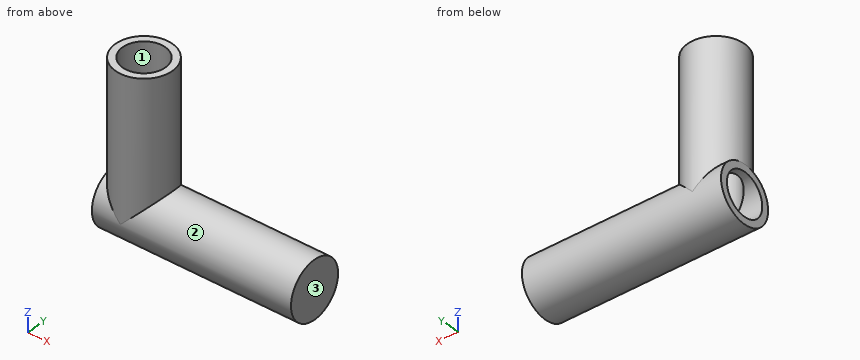
```python
from build123d import *

# Parameters (mm, degrees)
F0_R          = 10
F1_DEPTH      = 40
F1_DEPTH_BACK = 10
F2_R          = 10
F3_DEPTH      = 50
F3_DEPTH_BACK = 20
F4_R          = 7.5
F5_DEPTH      = 35
F5_DEPTH_BACK = 25
F6_R          = 7.5
F7_DEPTH      = 50


with BuildPart() as f1:
    # F0 (on Top) → F1 (new body, two sides)
    with BuildSketch(Plane.XY) as f1_sk:
        with Locations((-9.956808, 0)):
            Circle(F0_R)
    extrude(amount=F1_DEPTH)
    extrude(f1_sk.sketch, amount=-F1_DEPTH_BACK)

    # F2 (on Right) → F3 (join, two sides)
    with BuildSketch(Plane.YZ) as f3_sk:
        with Locations((0, -10)):
            Circle(F2_R)
    extrude(amount=F3_DEPTH)
    extrude(f3_sk.sketch, amount=-F3_DEPTH_BACK)

    # F4 (on Right) → F5 (cut, two sides)
    with BuildSketch(Plane.YZ) as f5_sk:
        with Locations((0, -10)):
            Circle(F4_R)
    extrude(amount=F5_DEPTH, mode=Mode.SUBTRACT)
    extrude(f5_sk.sketch, amount=-F5_DEPTH_BACK, mode=Mode.SUBTRACT)

    # F6 (on face) → F7 (cut)
    with BuildSketch(Plane.XY.offset(40)):
        with Locations((-9.956808, 0)):
            Circle(F6_R)
    extrude(amount=-F7_DEPTH, mode=Mode.SUBTRACT)


solid = f1.part
```
Model file for the job. Use its own axes, mm. Face numbers are marked on the shaded views. Give positions to 0.01 mm unless a question says otherwise; leave off trailing zeros. Loops run counter-clockwise (first coordinate to the right, second up) from the corner with the lowest first, then second, coordinate; pieces in that order, holes last. Notation, with made-up numbers: (50.5, 25) -> (88.5, 25) arc R18 ccw to (88.5, 32) -> close; hole circle Ø6 at (86, 79). An arc over 180 degrees is marked (long way). Write each question's results on one line, items separated by ' | '.
(1) Cut at D-D on y = -4.25. List the corners of the cut face in (x, z), and give its area (3 significant figures).
Geometry results:
outline: (-20, -19.05) -> (50, -19.05) -> (50, -0.95) -> (-0.9, -0.95) -> (-0.9, 40) -> (-3.78, 40) -> (-3.78, -3.82) -> (35, -3.82) -> (35, -16.18) -> (-20, -16.18) -> close; (-20, -3.82) -> (-16.14, -3.82) -> (-16.14, 40) -> (-19.01, 40) -> (-19.01, -0.95) -> (-20, -0.95) -> close | area: 787 mm²
(2) Probe line 1 along Z through (x, y) = (9, 0); line 2 along Y through (x, z) = (-15, -10); line 3 along X through (y, z) = (6, -13). List the from-to ranges inside material, lowest first.
Geometry results:
line 1: z = -20 to -17.5, -2.5 to 0 | line 2: y = -10 to -7.5, 7.5 to 10 | line 3: x = 35 to 50
(3) Pull direction Y, two halves, no side cores. Call the marked faces 1, 2 and 3: released by +Y, released by -Y, zero draft, split by the parting line, or undercut.
Geometry results:
face 1: undercut | face 2: split by the parting line | face 3: zero draft
(4) Cut at C-C on x = -11.5. List the corners of the cut face in (y, z).
Geometry results:
outline: (-9.88, -8.46) arc R10 ccw (long way) to (9.88, -8.46) -> (9.88, 40) -> (7.34, 40) -> (7.34, -8.46) arc R7.5 cw (long way) to (-7.34, -8.46) -> (-7.34, 40) -> (-9.88, 40) -> close
(5) Flat gauge pins, fed straight in: pin 1 Ø9 at (y, z) = (0, -10) entering from -X; pin 2 Ø12 at (x, y) = (13.5, -4.5) entering from -Z; pin 3 Ø3 at (x, y) = (19, 6.5) entering from -Z; pin 4 Ø6 at (y, z) = (-1.5, 5.5) entering from -X. Where does each tip first touch, or does it go through?
Geometry results:
pin 1: stops at x = 35 | pin 2: stops at z = -20 | pin 3: stops at z = -18.66 | pin 4: stops at x = -19.96
(6) Cut at B-B on z = -7.5. List the corners of the cut face in (x, y).
Geometry results:
outline: (-20, -9.68) -> (-12.46, -9.68) arc R10 ccw to (-7.46, -9.68) -> (50, -9.68) -> (50, 9.68) -> (-7.46, 9.68) arc R10 ccw to (-12.46, 9.68) -> (-20, 9.68) -> (-20, 7.07) -> (-12.46, 7.07) arc R7.5 cw to (-7.46, 7.07) -> (35, 7.07) -> (35, -7.07) -> (-7.46, -7.07) arc R7.5 cw to (-12.46, -7.07) -> (-20, -7.07) -> close
(7) Cut at A-A on y = 0. List the corners of the cut face in (x, z), and give its area (4 significant figures).
Geometry results:
outline: (-20, -20) -> (50, -20) -> (50, 0) -> (0.04, 0) -> (0.04, 40) -> (-2.46, 40) -> (-2.46, -2.5) -> (35, -2.5) -> (35, -17.5) -> (-20, -17.5) -> close; (-20, -2.5) -> (-17.46, -2.5) -> (-17.46, 40) -> (-19.96, 40) -> (-19.96, 0) -> (-20, 0) -> close | area: 737.5 mm²
